Design review of the part shown in the three views and the two pictorial views. Dimensions are in mm from the part's minimum x, y and z. Coordinates: 2 decimals unless noted, no trailing zeros. Write each loop counter-clockwise with the first axis right and the second up, starting at its lowest first coordinate (ties: lowest second). Pieces come first, ordered by that corner, then holes. Notation, with made-up numbers: (-36.5, -28.5) -> (-32.5, -28.5) arc R19 ccw to (-32.5, -18.5) -> close; hole circle Ø7 at (8, 3). An arc over 180 degrees is marked (long way). Write each question's results on one line, items separated by ' | '.
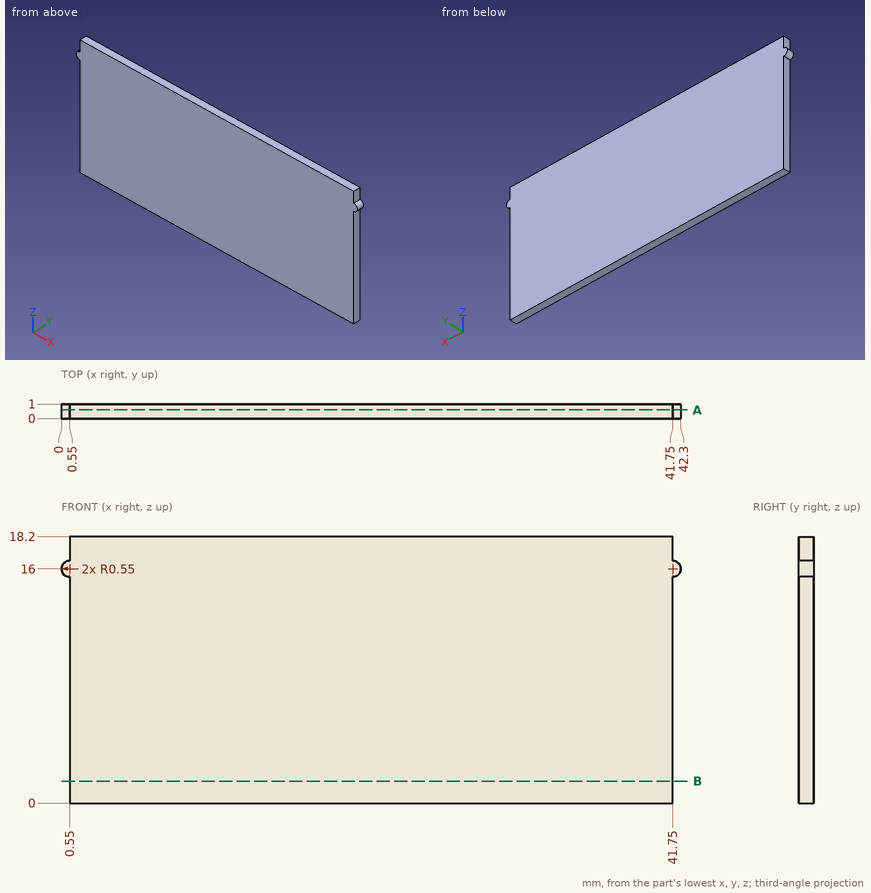
Q1. Clearance check with flat-ended pins moving along their axes: P1, Ø0.5, axis at y = 0.5, z = 8, coming from the -X side; P2, Ø0.5, axis at y = 0.5, z = 17.5, coming from the +X side. State where each tip first meets the part, or that it passes through.
Solution:
P1: x = 0.55 | P2: x = 41.75
Q2. Add section B-B (z = 1.5). Write out the cut boundary in (x, y).
Solution:
outline: (0.55, 0) -> (41.75, 0) -> (41.75, 1) -> (0.55, 1) -> close
Q3. For line 1 (X direction, y = 0.25, z = 13), list the stretches that pass through material, from the lowest coordinate up. Write a range as from..to.
Solution:
line 1: 0.55..41.75
Q4. Add section A-A (y = 0.6). Write out the cut boundary in (x, z), plus the area to 3 significant figures.
Solution:
outline: (0.55, 0) -> (41.75, 0) -> (41.75, 15.45) arc R0.55 ccw to (41.75, 16.55) -> (41.75, 18.2) -> (0.55, 18.2) -> (0.55, 16.55) arc R0.55 ccw to (0.55, 15.45) -> close | area: 751 mm²
